Input: part model. Units: mm. Frame: model coordinates. Face numbers are marked on the shaded views. A direction names the side the tool comes from. Give positions to 0.01 mm unless a question says otherwise; leave off trailing zeros. Loops run counter-clockwise (first coordinate to the right, second up) from the corner with the lowest first, then second, coordinate; pieces in that order, holes last. Notation, with made-up numbers: (-37.75, -1.5) -> (11.25, -1.5) arc R22 cw to (11.25, 10.5) -> close; hole circle Ø7 at (41, 64). An arc over 180 degrees is marked (long way). Answer as a JSON object with one key per item and string values.
```python
from build123d import *

# Parameters (mm, degrees)
F1_DEPTH      = 2.2
F2_DEPTH      = 4
F3_DEPTH      = 8
F5_W          = 4.721
F5_H          = 0.5
F6_DEPTH      = 2
F6_DEPTH_BACK = 10
F7_DEPTH      = 4
F8_T1_DEPTH   = 5.9270831351
F8_T3_DEPTH   = 8.1
F8_T5_DEPTH   = 4.721
F8_T11_DEPTH  = 12.0188296006
F8_T16_DEPTH  = 14.5648341529
F8_T24_DEPTH  = 14.5648341529
F8_T29_DEPTH  = 12.0188296006
F10_DEPTH     = 1.5
F12_DEPTH     = 2
F13_R         = 1


# Not quite as in the source:
# - a fillet or chamfer that OpenCascade refuses, or shapes differently, is made with other operations: its cross-section is extruded or revolved along the edge and cut away or added


with BuildPart() as f1:
    # F0 (on Front) → F1 (new body)
    with BuildSketch(Plane.XZ):
        with BuildLine():
            Line((-1.6440981598, 0.625), (-5.6, 0.625))
            Line((-5.6, 0.625), (-5.6, -0.625))
            Line((-5.6, -0.625), (-1.6440981598, -0.625))
            ThreePointArc((-1.6440981598, -0.625), (-1.6599999508, 0), (-1.6440981598, 0.625))
        make_face()
        with BuildLine():
            Line((-1.23, 0.625), (-1.6440981598, 0.625))
            ThreePointArc((-1.6440981598, 0.625), (-1.6599999508, 0), (-1.6440981598, -0.625))
            Line((-1.6440981598, -0.625), (-1.23, -0.625))
            Line((-1.23, -0.625), (1.2508001143, -0.625))
            ThreePointArc((1.2508001143, -0.625), (1.23, 0), (1.2508001143, 0.625))
            Line((1.2508001143, 0.625), (-1.23, 0.625))
        make_face()
        with BuildLine():
            Line((1.6420518568, 0.625), (1.2508001143, 0.625))
            ThreePointArc((1.2508001143, 0.625), (1.23, 0), (1.2508001143, -0.625))
            Line((1.2508001143, -0.625), (1.6420518568, -0.625))
            Line((1.6420518568, -0.625), (5.6, -0.625))
            Line((5.6, -0.625), (5.6, 0.625))
            Line((5.6, 0.625), (1.6420518568, 0.625))
        make_face()
    extrude(amount=F1_DEPTH)

    # F0 (on Front) → F2 (join)
    with BuildSketch(Plane.XZ):
        with BuildLine():
            Line((5.6, -2.8), (1.6566885771, -2.8))
            ThreePointArc((1.6566885771, -2.8), (1.8795878526, -3.4337692421), (2.1471830551, -4.05))
            Line((2.1471830551, -4.05), (5.6, -4.05))
            Line((5.6, -4.05), (5.6, -2.8))
        make_face()
        with BuildLine():
            Line((-1.23, -2.8), (-1.3368015602, -2.8))
            ThreePointArc((-1.3368015602, -2.8), (-1.1717307029, -3.4298126738), (-0.9735386938, -4.05))
            Line((-0.9735386938, -4.05), (0.8789681604, -4.05))
            Line((0.8789681604, -4.05), (2.1471830551, -4.05))
            ThreePointArc((2.1471830551, -4.05), (1.8795878526, -3.4337692421), (1.6566885771, -2.8))
            Line((1.6566885771, -2.8), (1.23, -2.8))
            Line((1.23, -2.8), (-1.23, -2.8))
        make_face()
        with BuildLine():
            Line((-1.735931594, -2.8), (-5.6, -2.8))
            Line((-5.6, -2.8), (-5.6, -4.05))
            Line((-5.6, -4.05), (-2.3307385194, -4.05))
            Line((-2.3307385194, -4.05), (-1.23, -4.05))
            Line((-1.23, -4.05), (-0.9735386938, -4.05))
            ThreePointArc((-0.9735386938, -4.05), (-1.1717307029, -3.4298126738), (-1.3368015602, -2.8))
            Line((-1.3368015602, -2.8), (-1.735931594, -2.8))
        make_face()
        Polygon((-7.1570831351, 4.05), (-5.6, 4.05), (-2.3307385194, 4.05), (-1.23, 4.05), (-1.23, 5.3), (-8.636245504, 5.3), (-8.636245504, -5.3), (-1.23, -5.3), (-1.23, -4.05), (-2.3307385194, -4.05), (-5.6, -4.05), (-7.1570831351, -4.05), align=None)
        Polygon((-5.6, -0.625), (-5.6, 0.625), (-5.6, 2.8), (-5.6, 4.05), (-7.1570831351, 4.05), (-7.1570831351, -4.05), (-5.6, -4.05), (-5.6, -2.8), align=None)
        with BuildLine():
            Line((-5.6, 4.05), (-5.6, 2.8))
            Line((-5.6, 2.8), (-1.735931594, 2.8))
            Line((-1.735931594, 2.8), (-1.3368015602, 2.8))
            ThreePointArc((-1.3368015602, 2.8), (-1.1717307029, 3.4298126738), (-0.9735386938, 4.05))
            Line((-0.9735386938, 4.05), (-1.23, 4.05))
            Line((-1.23, 4.05), (-2.3307385194, 4.05))
            Line((-2.3307385194, 4.05), (-5.6, 4.05))
        make_face()
        with BuildLine():
            ThreePointArc((-0.9735386938, 4.05), (-1.1717307029, 3.4298126738), (-1.3368015602, 2.8))
            Line((-1.3368015602, 2.8), (1.23, 2.8))
            Line((1.23, 2.8), (1.2939187969, 2.8))
            Line((1.2939187969, 2.8), (1.6566885771, 2.8))
            ThreePointArc((1.6566885771, 2.8), (1.8795878526, 3.4337692421), (2.1471830551, 4.05))
            Line((2.1471830551, 4.05), (0.8789681604, 4.05))
            Line((0.8789681604, 4.05), (-0.9735386938, 4.05))
        make_face()
        with BuildLine():
            ThreePointArc((2.1471830551, 4.05), (1.8795878526, 3.4337692421), (1.6566885771, 2.8))
            Line((1.6566885771, 2.8), (5.6, 2.8))
            Line((5.6, 2.8), (5.6, 4.05))
            Line((5.6, 4.05), (2.1471830551, 4.05))
        make_face()
    extrude(amount=F2_DEPTH)

    # F0 (on Front) → F3 (join)
    with BuildSketch(Plane.XZ):
        with BuildLine():
            ThreePointArc((2.1471830551, 4.05), (1.8795878526, 3.4337692421), (1.6566885771, 2.8))
            Line((1.6566885771, 2.8), (5.6, 2.8))
            Line((5.6, 2.8), (5.6, 4.05))
            Line((5.6, 4.05), (2.1471830551, 4.05))
        make_face()
        with BuildLine():
            Line((-5.6, 4.05), (-5.6, 2.8))
            Line((-5.6, 2.8), (-1.735931594, 2.8))
            Line((-1.735931594, 2.8), (-1.3368015602, 2.8))
            ThreePointArc((-1.3368015602, 2.8), (-1.1717307029, 3.4298126738), (-0.9735386938, 4.05))
            Line((-0.9735386938, 4.05), (-1.23, 4.05))
            Line((-1.23, 4.05), (-2.3307385194, 4.05))
            Line((-2.3307385194, 4.05), (-5.6, 4.05))
        make_face()
        Polygon((-5.6, -0.625), (-5.6, 0.625), (-5.6, 2.8), (-5.6, 4.05), (-7.1570831351, 4.05), (-7.1570831351, -4.05), (-5.6, -4.05), (-5.6, -2.8), align=None)
        with BuildLine():
            Line((-1.735931594, -2.8), (-5.6, -2.8))
            Line((-5.6, -2.8), (-5.6, -4.05))
            Line((-5.6, -4.05), (-2.3307385194, -4.05))
            Line((-2.3307385194, -4.05), (-1.23, -4.05))
            Line((-1.23, -4.05), (-0.9735386938, -4.05))
            ThreePointArc((-0.9735386938, -4.05), (-1.1717307029, -3.4298126738), (-1.3368015602, -2.8))
            Line((-1.3368015602, -2.8), (-1.735931594, -2.8))
        make_face()
        with BuildLine():
            Line((5.6, -2.8), (1.6566885771, -2.8))
            ThreePointArc((1.6566885771, -2.8), (1.8795878526, -3.4337692421), (2.1471830551, -4.05))
            Line((2.1471830551, -4.05), (5.6, -4.05))
            Line((5.6, -4.05), (5.6, -2.8))
        make_face()
    extrude(amount=F3_DEPTH)

    # F5 (on face) → F6 (join, two sides)
    with BuildSketch(Plane.XY.offset(4.05)) as f6_sk:
        with Locations((3.2395, -0.25)):
            Rectangle(F5_W, F5_H)
    extrude(amount=F6_DEPTH)
    extrude(f6_sk.sketch, amount=-F6_DEPTH_BACK)

    # F4 (on face) → F7 (cut)
    with BuildSketch(Plane(origin=(-8.636245504, 0, 0), x_dir=(0, -1, 0), z_dir=(-1, 0, 0))):
        with BuildLine():
            ThreePointArc((2.2, 0.625), (3.2875, 1.7125), (2.2, 2.8))
            Line((2.2, 2.8), (0, 2.8))
            Line((0, 2.8), (0, 0.625))
            Line((0, 0.625), (2.2, 0.625))
        make_face()
        with BuildLine():
            ThreePointArc((2.2659621103, -2.8), (3.3204810552, -1.6795189448), (2.2, -0.625))
            Line((2.2, -0.625), (0, -0.625))
            Line((0, -0.625), (0, -2.8))
            Line((0, -2.8), (2.2, -2.8))
            Line((2.2, -2.8), (2.2659621103, -2.8))
        make_face()
    extrude(amount=-F7_DEPTH, mode=Mode.SUBTRACT)

    # F8: fillet of radius 3 on 5 edges, made by hand

    # F8_s2 → F8_t1 (join)
    with BuildSketch(Plane.YZ.offset(-7.1570831351)):
        with BuildLine():
            ThreePointArc((-4, 5.3), (-5.0673921924, 4.380730437), (-6.4366985862, 4.05))
            Line((-6.4366985862, 4.05), (-4, 4.05))
            Line((-4, 4.05), (-4, 5.3))
        make_face()
        with BuildLine():
            ThreePointArc((-4, -5.3), (-5.0673921924, -4.380730437), (-6.4366985862, -4.05))
            Line((-6.4366985862, -4.05), (-4, -4.05))
            Line((-4, -4.05), (-4, -5.3))
        make_face()
    extrude(amount=F8_T1_DEPTH)

    # F8_s4 → F8_t3 (join)
    with BuildSketch(Plane.XY.offset(-4.05)):
        with BuildLine():
            ThreePointArc((-8.636245504, -4), (-7.5529985653, -5.0963889141), (-7.1570831351, -6.5859336612))
            Line((-7.1570831351, -6.5859336612), (-7.1570831351, -4))
            Line((-7.1570831351, -4), (-8.636245504, -4))
        make_face()
    extrude(amount=F8_T3_DEPTH)

    # F8_s6 → F8_t5 (join)
    with BuildSketch(Plane.YZ.offset(0.879)):
        with BuildLine():
            ThreePointArc((-0.5, -5.95), (-1.6028628458, -4.5700806465), (-3.2910571474, -4.05))
            Line((-3.2910571474, -4.05), (-0.5, -4.05))
            Line((-0.5, -4.05), (-0.5, -5.95))
        make_face()
        with BuildLine():
            ThreePointArc((-0.5, 6.05), (-1.5963763172, 4.6005102572), (-3.3284271247, 4.05))
            Line((-3.3284271247, 4.05), (-0.5, 4.05))
            Line((-0.5, 4.05), (-0.5, 6.05))
        make_face()
    extrude(amount=F8_T5_DEPTH)


with BuildPart() as f8_tool9:
    # F8_s10 → F8_t11 (new body)
    with BuildSketch(Plane.YZ.offset(-13.2488296006)):
        with BuildLine():
            ThreePointArc((-4, 5.3), (-5.0673921924, 4.380730437), (-6.4366985862, 4.05))
            Line((-6.4366985862, 4.05), (-4, 4.05))
            Line((-4, 4.05), (-4, 5.3))
        make_face()
    extrude(amount=F8_T11_DEPTH)

    split(bisect_by=Plane.YZ.offset(-7.1570831351), keep=Keep.BOTTOM)

    split(bisect_by=Plane.YZ.offset(-8.636245504), keep=Keep.TOP)


with BuildPart() as f8_tool14:
    # F8_s15 → F8_t16 (new body)
    with BuildSketch(Plane.XY.offset(-4.05)):
        with BuildLine():
            ThreePointArc((-8.636245504, -4), (-7.5529985653, -5.0963889141), (-7.1570831351, -6.5859336612))
            Line((-7.1570831351, -6.5859336612), (-7.1570831351, -4))
            Line((-7.1570831351, -4), (-8.636245504, -4))
        make_face()
    extrude(amount=F8_T16_DEPTH)

    split(bisect_by=Plane.XY.offset(5.3), keep=Keep.BOTTOM)

    split(bisect_by=Plane.XY.offset(4.05), keep=Keep.TOP)


with BuildPart() as f8_tool9_1:
    add(f8_tool9.part)

    # F8_t19: intersect F8_tool14
    add(f8_tool14.part, mode=Mode.INTERSECT)


with BuildPart() as f1_1:
    add(f1.part)

    # F8_t7: union F8_tool9
    add(f8_tool9_1.part)


with BuildPart() as f8_tool22:
    # F8_s23 → F8_t24 (new body)
    with BuildSketch(Plane.XY.offset(-10.5148341529)):
        with BuildLine():
            ThreePointArc((-8.636245504, -4), (-7.5529985653, -5.0963889141), (-7.1570831351, -6.5859336612))
            Line((-7.1570831351, -6.5859336612), (-7.1570831351, -4))
            Line((-7.1570831351, -4), (-8.636245504, -4))
        make_face()
    extrude(amount=F8_T24_DEPTH)

    split(bisect_by=Plane.XY.offset(-5.3), keep=Keep.TOP)

    split(bisect_by=Plane.XY.offset(-4.05), keep=Keep.BOTTOM)


with BuildPart() as f8_tool27:
    # F8_s28 → F8_t29 (new body)
    with BuildSketch(Plane.YZ.offset(-1.23)):
        with BuildLine():
            ThreePointArc((-4, -5.3), (-5.0673921924, -4.380730437), (-6.4366985862, -4.05))
            Line((-6.4366985862, -4.05), (-4, -4.05))
            Line((-4, -4.05), (-4, -5.3))
        make_face()
    extrude(amount=-F8_T29_DEPTH)

    split(bisect_by=Plane.YZ.offset(-7.1570831351), keep=Keep.BOTTOM)

    split(bisect_by=Plane.YZ.offset(-8.636245504), keep=Keep.TOP)


with BuildPart() as f8_tool22_1:
    add(f8_tool22.part)

    # F8_t32: intersect F8_tool27
    add(f8_tool27.part, mode=Mode.INTERSECT)


with BuildPart() as f1_2:
    add(f1_1.part)

    # F8_t20: union F8_tool22
    add(f8_tool22_1.part)

    # F9 (on face) → F10 (cut)
    with BuildSketch(Plane.XY.offset(4.05)):
        with BuildLine():
            Line((-1.23, 0), (-1.23, -2.1719092038))
            ThreePointArc((-1.23, -2.1719092038), (-0.1755, -2.7577127774), (0.879, -2.1719092038))
            Line((0.879, -2.1719092038), (0.879, 0))
            Line((0.879, 0), (-1.23, 0))
        make_face()
    extrude(amount=-F10_DEPTH, mode=Mode.SUBTRACT)

    # F11 (on face) → F12 (cut)
    with BuildSketch(Plane(origin=(0, 0, -4.05), x_dir=(1, 0, 0), z_dir=(0, 0, -1))):
        with BuildLine():
            ThreePointArc((0.879, 2.1719092038), (-0.1755, 2.7577127774), (-1.23, 2.1719092038))
            Line((-1.23, 2.1719092038), (-1.23, 0))
            Line((-1.23, 0), (0.879, 0))
            Line((0.879, 0), (0.879, 0.5))
            Line((0.879, 0.5), (0.879, 2.1719092038))
        make_face()
    extrude(amount=-F12_DEPTH, mode=Mode.SUBTRACT)

    # F13
    f13_edges = [f1_2.edges().sort_by_distance(p)[0] for p in [
        (-4.065311, -8, 4.05),
        (-7.157083, -8, 0),
        (-4.065311, -8, -4.05),
        (3.873592, -8, -4.05),
        (3.873592, -8, 4.05),
    ]]
    fillet(f13_edges, radius=F13_R)


solid = f1_2.part
```
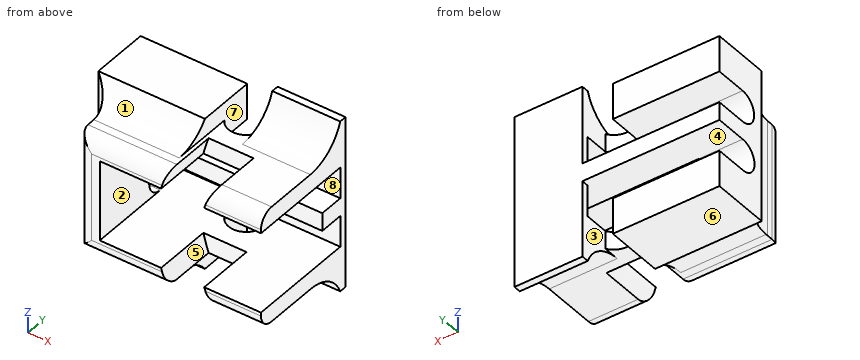
Q1. Ray query, line 1 along Z through (x, y) = (-5.25, -0.75) (3 decimals); line 2 along Z through (x, y) = (-3, -7); line 3 along X through (y, z) = (-1.25, -4.5). Return the intervals inside material, ascending.
Evaluation:
{"line 1": "z = -5.3 to -2.8, -0.625 to 0.625, 2.8 to 5.3", "line 2": "z = -4.05 to -2.8, 2.8 to 4.05", "line 3": "x = -8.64 to -1.23, 0.88 to 5.6"}
Q2. Access query for the marked faces 5, 6, 7 and 8. Directions: +Z, -Z, +X, -X, +Y, -Y. A direction counts if a zero-diameter tool reaches every point of the face in a straight line with its end or side. Return the directions, or none.
Evaluation:
{"face 5": "-Y", "face 6": "-Z, -X, +Y, -Y", "face 7": "+Z, +Y", "face 8": "+X, -X, -Y"}
Q3. Section A-A, the plane x = -5.25. Return the cut outline in (y, z) (3 decimals).
Evaluation:
{"outline": "(-8, -3.05) arc R1 ccw to (-7, -4.05) -> (-6.437, -4.05) arc R3 cw to (-4, -5.3) -> (0, -5.3) -> (0, -2.8) -> (-8, -2.8) -> close; (-8, 2.8) -> (0, 2.8) -> (0, 5.3) -> (-4, 5.3) arc R3 cw to (-6.437, 4.05) -> (-7, 4.05) arc R1 ccw to (-8, 3.05) -> close; (-2.2, -0.625) -> (0, -0.625) -> (0, 0.625) -> (-2.2, 0.625) -> close"}
Q4. Section C-C, the plane y = -5. Return the cut outline in (x, z), then the cut area to 3 significant figures.
Evaluation:
{"outline": "(-7.61, -4.42) -> (-1.23, -4.42) -> (-1.23, -4.05) -> (-0.97, -4.05) arc R12.29 cw to (-1.34, -2.8) -> (-5.6, -2.8) -> (-5.6, 2.8) -> (-1.34, 2.8) arc R12.29 cw to (-0.97, 4.05) -> (-1.23, 4.05) -> (-1.23, 4.42) -> (-7.61, 4.42) -> close; (1.66, -2.8) arc R9.4 ccw to (2.15, -4.05) -> (5.6, -4.05) -> (5.6, -2.8) -> close; (1.66, 2.8) -> (5.6, 2.8) -> (5.6, 4.05) -> (2.15, 4.05) arc R9.4 ccw to start", "area": "41.3 mm2"}
Q5. Section D-D, the plane x = -0.25. Return the cut outline in (y, z) (3 decimals), then the cut area to 3 significant figures.
Evaluation:
{"outline": "(-4, -4.05) -> (-2.755, -4.05) -> (-2.755, -2.8) -> (-4, -2.8) -> close; (-4, 2.8) -> (-2.755, 2.8) -> (-2.755, 4.05) -> (-4, 4.05) -> close; (-2.2, -0.625) -> (0, -0.625) -> (0, 0.625) -> (-2.2, 0.625) -> close", "area": "5.86 mm2"}
Q6. Pin query (flat end, axial travel): pin 1 (1.4 mm diameter, centred on x = 0, z = -3.5, fed in from -Y); pin 2 (2 mm diameter, centred on x = -4, z = 1, fed in from -Y); pin 3 (1.2 mm diameter, centred on x = -3.5, y = -2, fed in from +Z). Return the tip coordinate at first contact, or that it passes through.
Evaluation:
{"pin 1": "stops at y = -4", "pin 2": "stops at y = -2.2", "pin 3": "stops at z = 5.3"}
Q7. Draft query along Z for the marked faces 1, 2, 3 and 4. Return one class per face: +Z half, -Z half, draft (parallel to the pull), parting line (faces both ways), or undercut.
Evaluation:
{"face 1": "+Z half", "face 2": "undercut", "face 3": "draft", "face 4": "undercut"}
Q8. Section B-B, the plane z = 2.5. Return the cut outline in (x, y).
Evaluation:
{"outline": "(-8.64, -4) arc R3 cw to (-7.16, -6.59) -> (-7.16, -7) arc R1 ccw to (-6.16, -8) -> (-5.6, -8) -> (-5.6, -2.95) -> (-8.64, -2.95) -> close; (0.88, -0.5) -> (5.6, -0.5) -> (5.6, 0) -> (0.88, 0) -> close"}
